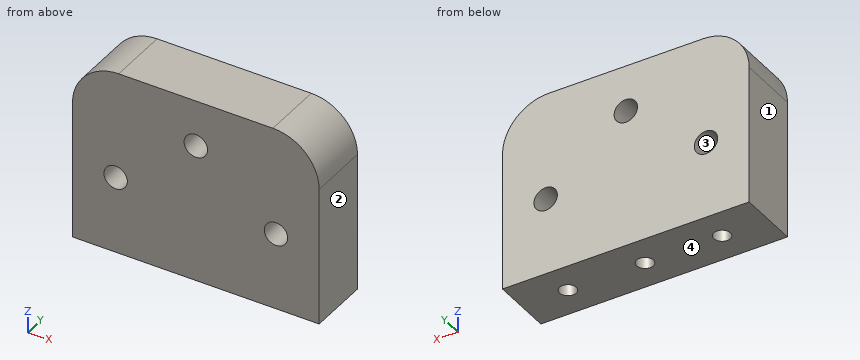
from build123d import *

# Parameters (mm, degrees)
BOSS_EXTRUDE1_DEPTH       = 10
F_6_CLEARANCE_HOLE1_D     = 3.7973
F_6_32_TAPPED_HOLE1_D     = 2.7051
F_6_32_TAPPED_HOLE1_DEPTH = 9.53
F_6_32_TAPPED_HOLE1_TIP   = 0.81269403


with BuildPart() as part:
    # Sketch1 → Boss-Extrude1 (new body)
    with BuildSketch(Plane(origin=(0, 0, 0), x_dir=(1, 0, 0), z_dir=(0, 1, 0))):
        with BuildLine():
            Line((0, 0), (40, 0))
            Line((40, 0), (40, -22.5))
            ThreePointArc((40, -22.5), (37.803300859, -27.803300859), (32.5, -30))
            Line((32.5, -30), (7.5, -30))
            ThreePointArc((7.5, -30), (2.196699141, -27.803300859), (0, -22.5))
            Line((0, -22.5), (0, 0))
        make_face()
    extrude(amount=BOSS_EXTRUDE1_DEPTH)

    # #6 Clearance Hole1 (through all)
    with Locations(Plane(origin=(0, 10, 0), x_dir=(1, 0, 0), z_dir=(0, 1, 0))):
        with Locations((7, -12.5), (33, -12.5), (20, -22.5)):
            Hole(F_6_CLEARANCE_HOLE1_D / 2)

    # #6-32 Tapped Hole1
    with Locations(Plane(origin=(0, 0, 0), x_dir=(-1, 0, 0), z_dir=(0, 0, -1))):
        with Locations((-32.5, 5), (-20, 5), (-7.5, 5)):
            Hole(F_6_32_TAPPED_HOLE1_D / 2, depth=F_6_32_TAPPED_HOLE1_DEPTH)
            with Locations((0, 0, -(F_6_32_TAPPED_HOLE1_DEPTH + F_6_32_TAPPED_HOLE1_TIP / 2))):  # 118° drill point
                Cone(0, F_6_32_TAPPED_HOLE1_D / 2, F_6_32_TAPPED_HOLE1_TIP, mode=Mode.SUBTRACT)


solid = part.part
Geometry: final body of the model. Coordinates: model frame, mm. Face numbers are marked on the shaded views. Round coordinates to 2 decimals unless told otherwise and drop trailing zeros. Order: outer loops, then holes, each group sorted by start corner. A loop starts at its lowest first (then second) coordinate and runs counter-clockwise, first axis right, second up. Notation, with made-up numbers: (78.5, -29) - (82.5, -29) arc R7 ccw to (82.5, -17) - close; hole circle Ø9 at (-35.5, -15). An arc over 180 degrees is marked (long way). Write each question's results on one line, items separated by ' | '.
Item 1: Section D-D, the plane x = 3. Return the cut outline in (y, z), and give its area (3 significant figures).
Completed:
outline: (0, 0) - (10, 0) - (10, 28.5) - (0, 28.5) - close | area: 285 mm^2
Item 2: Section C-C, the plane y = 8. Return the cut outline in (x, z), and give its area (3 significant figures).
Completed:
outline: (0, 0) - (40, 0) - (40, 22.5) arc R7.5 ccw to (32.5, 30) - (7.5, 30) arc R7.5 ccw to (0, 22.5) - close; hole circle Ø3.8 at (7, 12.5); hole circle Ø3.8 at (20, 22.5); hole circle Ø3.8 at (33, 12.5) | area: 1,140 mm^2
Item 3: Mould query, pull axis X, two halves, no side actions, for the marked faces 1, 2, 3 and 4. Classes: pulls with the +X half, pulls with the -X half, needs draft (parallel to the pull), parting line crosses it, or undercut.
Completed:
face 1: pulls with the -X half | face 2: pulls with the +X half | face 3: undercut | face 4: needs draft
Item 4: Section B-B, the plane z = 9. Return the cut outline in (x, y), and give its area (3 significant figures).
Completed:
outline: (0, 0) - (40, 0) - (40, 10) - (0, 10) - close; hole circle Ø2.71 at (7.5, 5); hole circle Ø2.71 at (20, 5); hole circle Ø2.71 at (32.5, 5) | area: 383 mm^2
Item 5: First-contact query: pin 1 Ø3 at (x, z) = (7, 12.5) entering from -Y; pin 2 Ø1.5 at (y, z) = (8.5, 26) entering from +X; pin 3 Ø2 at (x, y) = (32.5, 5) entering from -Z. Flat tips, straight axial feed; report the tip coordinate or a pass-through.
Completed:
pin 1: through | pin 2: x = 39.48 | pin 3: z = 9.74
Item 6: Material intervals for line 1 along X through (y, z) = (5, 3); line 2 along Z through (x, y) = (20, 3); line 3 along X through (y, z) = (3, 12.5), sorted ascending. Write a range as [from, to].
Completed:
line 1: [0, 6.15], [8.85, 18.65], [21.35, 31.15], [33.85, 40] | line 2: [0, 20.6], [24.4, 30] | line 3: [0, 5.1], [8.9, 31.1], [34.9, 40]
Item 7: Section A-A, the plane z = 12.5. Return the cut outline in (x, y).
Completed:
outline: (0, 0) - (5.1, 0) - (5.1, 10) - (0, 10) - close; (8.9, 0) - (31.1, 0) - (31.1, 10) - (8.9, 10) - close; (34.9, 0) - (40, 0) - (40, 10) - (34.9, 10) - close
